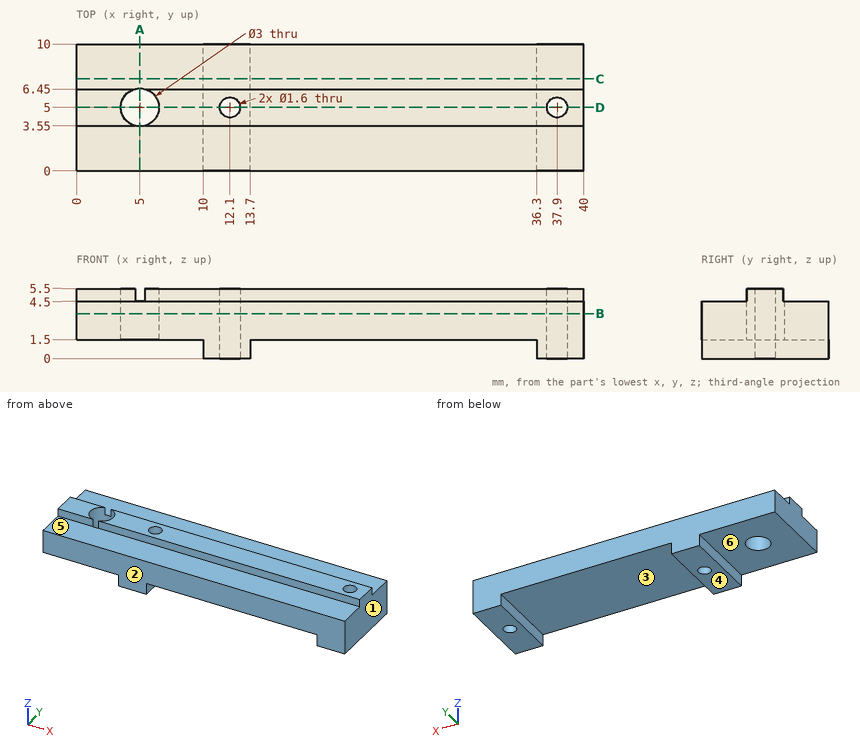
Check sheet for the drawn part. Datum: minimum x, y, z corner. Units: mm. A direction names the side the tool comes from. Round coordinates to 2 decimals unless told otherwise and drop trailing zeros. Loops run counter-clockwise (first coordinate to the right, second up) from the corner with the lowest first, then second, coordinate; pieces in that order, holes last. Notation, with made-up numbers: (87.25, 28) - (129.25, 28) arc R26 ccw to (129.25, 58) - close; hole circle Ø3 at (57.5, 41.25). An arc over 180 degrees is marked (long way). Write item = value, one per line. Start each with the question number.
1. Depth check by flat-ended pin: pin 1 (0.5 mm diameter, centred on x = 2, z = 5, fed in from -Y); pin 2 (1.6 mm diameter, centred on y = 6, z = 1, fed in from -X); pin 3 (1.2 mm diameter, centred on y = 4.5, z = 0.5, fed in from -X); pin 4 (3 mm diameter, centred on x = 22, y = 8, fed in from +Z). Enter the tip coordinate at first touch or a pass-through.
2. Thickness scan on line 1 (Y direction, x = 5, z = 3.95); line 2 (X direction, y = 8.5, z = 1.2); line 3 (X direction, y = 5.25, z = 1.35). Record the ranges inside material, lowest first.
3. Set-up check for the marked faces 4, 5 and 6: record each of +Z, -Z, +X, -X, +Y, -Y from which the full face is reachable in a straight line by a thin tool's end or side.
4. Section check A-A on x = 5. Enter the section's corners in (y, z), then the cut area to 3 significant figures.
5. Section check C-C on y = 7.25. Enter the section's corners in (x, z), then the cut area to 3 significant figures.
6. Mould release check, pull along X, two halves, no side actions. Record for the marked faces 1, 2 and 3: released by +X, released by -X, zero draft, split by the parting line, or undercut.
7. Section check D-D on y = 5. Enter the section's corners in (x, z), then the cut area to 4 significant figures.
8. Section check B-B on z = 3.55. Enter the section's corners in (x, y), then the cut area to 3 significant figures.
Working result:
q1.pin_1 = 3.55
q1.pin_2 = 0
q1.pin_3 = 10
q1.pin_4 = 4.5
q2.line_1 = 0 to 3.5, 6.5 to 10
q2.line_2 = 10 to 13.7, 36.3 to 40
q2.line_3 = 10 to 11.34, 12.86 to 13.7, 36.3 to 37.14, 38.66 to 40
q3.face_4 = -Z, +X, -X, +Y, -Y
q3.face_5 = +Z, +X, -X, -Y
q3.face_6 = -Z, -X, +Y, -Y
q4.outline = (0, 1.5) - (3.5, 1.5) - (3.5, 4.5) - (0, 4.5) - close; (6.5, 1.5) - (10, 1.5) - (10, 4.5) - (6.5, 4.5) - close
q4.area = 21.0 mm^2
q5.outline = (0, 1.5) - (10, 1.5) - (10, 0) - (13.7, 0) - (13.7, 1.5) - (36.3, 1.5) - (36.3, 0) - (40, 0) - (40, 4.5) - (0, 4.5) - close
q5.area = 131 mm^2
q6.face_1 = released by +X
q6.face_2 = zero draft
q6.face_3 = undercut
q7.outline = (0, 1.5) - (3.5, 1.5) - (3.5, 5.5) - (0, 5.5) - close; (6.5, 1.5) - (10, 1.5) - (10, 0) - (11.3, 0) - (11.3, 5.5) - (6.5, 5.5) - close; (12.9, 0) - (13.7, 0) - (13.7, 1.5) - (36.3, 1.5) - (36.3, 0) - (37.1, 0) - (37.1, 5.5) - (12.9, 5.5) - close; (38.7, 0) - (40, 0) - (40, 5.5) - (38.7, 5.5) - close
q7.area = 141.5 mm^2
q8.outline = (0, 0) - (40, 0) - (40, 10) - (0, 10) - close; hole circle Ø3 at (5, 5); hole circle Ø1.6 at (12.1, 5); hole circle Ø1.6 at (37.9, 5)
q8.area = 389 mm^2
